Design review of the part shown in the three views and the two pictorial views. Dimensions are in mm from the part's minimum x, y and z. A direction names the side the tool comes from. Give positions to 0.01 mm unless a question says otherwise; leave off trailing zeros. Write each loop counter-clockwise with the first axis right and the second up, starting at its lowest first coordinate (ties: lowest second). Pieces come first, ordered by that corner, then holes. Notation, with made-up numbers: M -38.5,12.5 L 17.5,12.5 A25 ccw 17.5,41.5 Z; hole C 1,-26.5 d2. An arc over 180 degrees is marked long. Write item = value, one per line.
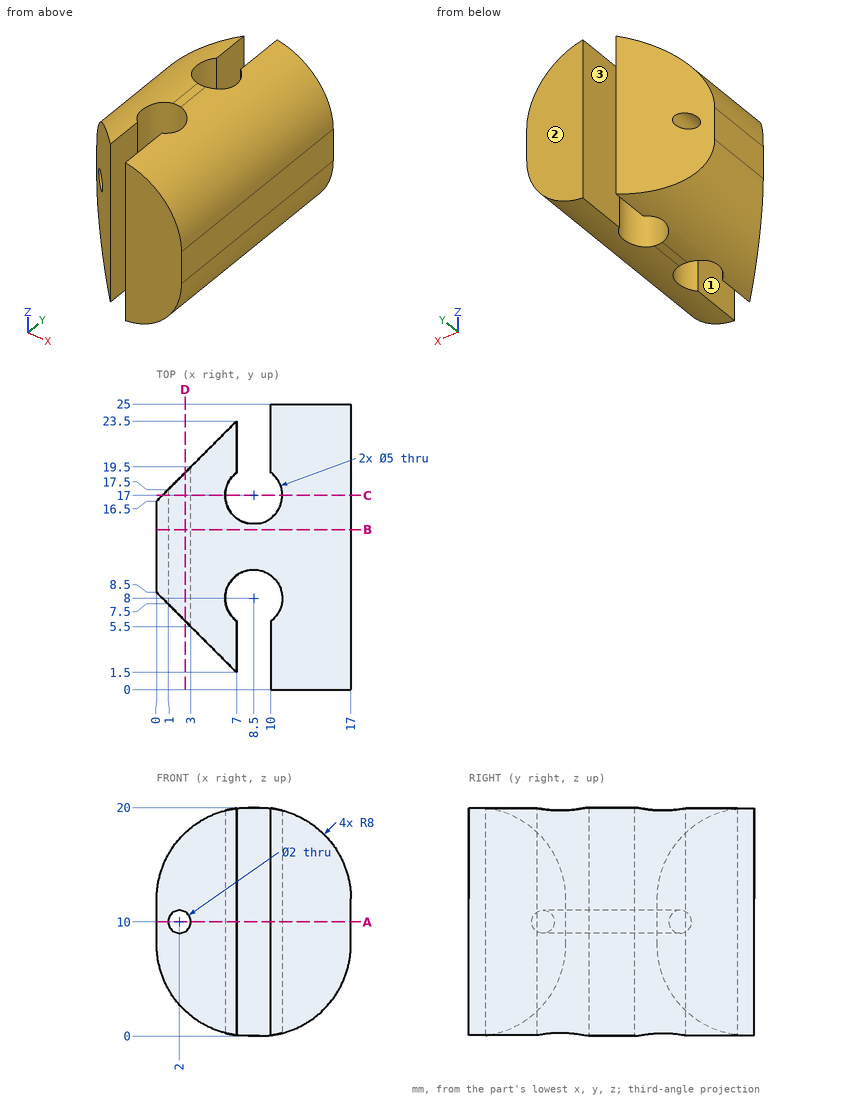
1. Machinability: for the marked faces 1, 2 and 3, which of the approach directions +Z, -Z, +X, -X, +Y, -Y give a long, thin tool a straight path to every point of the face, cutting with its end or side? Answer none if there is none.
Responses:
face_1 = +Z, -Z, -Y
face_2 = +Z, -Z, +X, -X, +Y
face_3 = +Z, -Z, +Y
2. For line 1 along X through (y, z) = (22, 10.25); line 2 along X through (y, z) = (8, 13.25); line 3 along Y through (x, z) = (10.75, 2.5), list the stretches that pass through material, from the lowest coordinate up. Write a range as from..to.
Responses:
line_1 = 5.5..7, 10..17
line_2 = 0.5..6, 11..16.9
line_3 = 0..6.91, 9.09..15.91, 18.09..25
3. We need section A-A, the plane z = 10. Write out the cut boundary in (x, y), then the cut area to 3 significant figures.
Responses:
outline = M 0,8.5 L 1,7.5 L 1,17.5 L 0,16.5 Z; M 3,5.5 L 7,1.5 L 7,6 A2.5 cw long 10,6 L 10,0 L 17,0 L 17,25 L 10,25 L 10,19 A2.5 cw long 7,19 L 7,23.5 L 3,19.5 Z
area = 258 mm2
4. Insertion check: P1, Ø5, axis at y = 21, z = 14.5, coming from the +X side; P2, Ø5, axis at y = 23, z = 6, coming from the -X side; P3, Ø5, axis at y = 3.5, z = 9, coming from the -X side; P4, Ø3, axis at x = 4, z = 11, coming from the -Y side. Each pin has a flat end and moves straight along its axis. Give the tip position at first contact, or say it passes through.
Responses:
P1 = 17
P2 = 4
P3 = 2.5
P4 = 3
5. We need section C-C, the plane y = 17. Write out the cut boundary in (x, z), then the cut area to 3 significant figures.
Responses:
outline = M 0.5,5.22 A8 ccw 6,0.25 L 6,19.75 A8 ccw 0.5,14.78 Z; M 11,0.25 A8 ccw 17,8 L 17,12 A8 ccw 11,19.75 Z; hole C 2,10 d2
area = 179 mm2
6. We need section D-D, the plane x = 2.5. Write out the cut boundary in (y, z), then the cut area to 3 significant figures.
Responses:
outline = M 6,2.19 L 19,2.19 L 19,9.13 L 6,9.13 Z; M 6,10.87 L 19,10.87 L 19,17.81 L 6,17.81 Z
area = 181 mm2
7. We need section B-B, the plane y = 14. Write out the cut boundary in (x, z).
Responses:
outline = M 0,8 A8 ccw 8,0 L 9,0 A8 ccw 17,8 L 17,12 A8 ccw 9,20 L 8,20 A8 ccw 0,12 Z; hole C 2,10 d2
